Verification items for the finished model (mm, model axes). A direction names the side the tool comes from. Give positions to 0.01 mm unless a question says otherwise; leave off trailing zeros. Write each loop counter-clockwise with the first axis right and the second up, starting at its lowest first coordinate (ties: lowest second). Pieces come first, ordered by that corner, then holes. Notation, with made-up numbers: (-20, 22.5) - (-1, 22.5) arc R18 ccw to (-1, 45.5) - close; hole circle Ø11 at (23.25, 16.25). An arc over 180 degrees is marked (long way). Put each result on its own line as item: value.
Autodesk Inventor part; units mm, degrees
ref_plane "GUS_4500_1_XY" through (7.5, 20, 0) normal (1, 0, 0) x (0, 0, -1)
ref_plane "GUS_4500_1_YZ" through (7.5, 20, 0) normal (0, 0, -1) x (0, 1, 0)
ref_plane "GUS_4500_1_ZX" through (7.5, 20, 0) normal (0, 1, 0) x (1, 0, 0)
sketch "Skizze_1" plane through (0, 0, 0) normal (0, 0, 1) x (1, 0, 0)
  line L0 (0, 0) -> (40, 0)
  line L1 (40, 0) -> (40, 5.8)
  line L2 (40, 5.8) -> (18.3181, 18.3181)
  line L3 (18.3181, 18.3181) -> (5.8, 40)
  line L4 (5.8, 40) -> (0, 40)
  line L5 (0, 40) -> (0, 0)
extrude "Extrusion1" add sketch "Skizze_1" along normal mid plane 37
sketch "Skizze_2" plane through (0, 0, 0) normal (0, 0, 1) x (1, 0, 0)
  line L0 (7.5, 7.5) -> (40, 7.5)
  line L1 (40, 7.5) -> (40, 40)
  line L2 (40, 40) -> (7.5, 40)
  line L3 (7.5, 40) -> (7.5, 7.5)
extrude "Extrusion2" cut sketch "Skizze_2" along normal mid plane 25
sketch "Skizze_3" plane through (0, 0, 0) normal (0, 1, 0) x (-1, 0, 0)
  arc A0 (-20.3, -4.5) -> (-20.3, 4.5) centre (-20.3, 0) ccw
  line L0 (-20.3, 4.5) -> (-25.3, 4.5)
  arc A1 (-25.3, 4.5) -> (-25.3, -4.5) centre (-25.3, 0) ccw
  line L1 (-25.3, -4.5) -> (-20.3, -4.5)
extrude "Extrusion3" cut sketch "Skizze_3" along normal blind 7.5
sketch "Skizze_4" plane through (0, 0, 0) normal (1, 0, 0) x (0, 1, 0)
  arc A0 (20.3, 4.5) -> (20.3, -4.5) centre (20.3, 0) ccw
  line L0 (20.3, -4.5) -> (25.3, -4.5)
  arc A1 (25.3, -4.5) -> (25.3, 4.5) centre (25.3, 0) ccw
  line L1 (25.3, 4.5) -> (20.3, 4.5)
extrude "Extrusion4" cut sketch "Skizze_4" along normal blind 7.5
sketch "Skizze_5" plane through (0, 0, 0) normal (1, 0, 0) x (0, 1, 0)
  line L0 (13, 7) -> (13, -7)
  line L1 (13, -7) -> (32, -7)
  line L2 (32, -7) -> (32, 7)
  line L3 (32, 7) -> (13, 7)
extrude "Extrusion5" cut sketch "Skizze_5" along normal blind 2
sketch "Skizze_6" plane through (0, 0, 0) normal (0, 1, 0) x (-1, 0, 0)
  line L0 (-13, 7) -> (-32, 7)
  line L1 (-32, 7) -> (-32, -7)
  line L2 (-32, -7) -> (-13, -7)
  line L3 (-13, -7) -> (-13, 7)
extrude "Extrusion6" cut sketch "Skizze_6" along normal blind 2
ref_plane "GUS_4500_1_XY" through (7.5, 20, 0) normal (1, 0, 0) x (0, 0, -1)
ref_plane "GUS_4500_1_YZ" through (7.5, 20, 0) normal (0, 0, -1) x (0, 1, 0)
ref_plane "GUS_4500_1_ZX" through (7.5, 20, 0) normal (0, 1, 0) x (1, 0, 0)
ref_plane "GUS_4500_12_XY" through (7.5, 25, 0) normal (1, 0, 0) x (0, 0, -1)
ref_plane "GUS_4500_12_YZ" through (7.5, 25, 0) normal (0, 0, -1) x (0, 1, 0)
ref_plane "GUS_4500_12_ZX" through (7.5, 25, 0) normal (0, 1, 0) x (1, 0, 0)
ref_plane "GUS_4500_2_XY" through (25, 7.5, 0) normal (0, 1, 0) x (1, 0, 0)
ref_plane "GUS_4500_2_YZ" through (25, 7.5, 0) normal (1, 0, 0) x (0, 0, -1)
ref_plane "GUS_4500_2_ZX" through (25, 7.5, 0) normal (0, 0, -1) x (0, 1, 0)
ref_plane "GUS_4500_23_XY" through (20, 7.5, 0) normal (0, 1, 0) x (1, 0, 0)
ref_plane "GUS_4500_23_YZ" through (20, 7.5, 0) normal (1, 0, 0) x (0, 0, -1)
ref_plane "GUS_4500_23_ZX" through (20, 7.5, 0) normal (0, 0, -1) x (0, 1, 0)
ref_plane "p1_XY" through (0, 20, -18.5) normal (0, 0, -1) x (0, 1, 0)
ref_plane "p1_YZ" through (0, 20, -18.5) normal (0, 1, 0) x (1, 0, 0)
ref_plane "p1_ZX" through (0, 20, -18.5) normal (1, 0, 0) x (0, 0, -1)
properties part number "GUS_4501_1"
Q1. Section check A-A, the plane y = 3.5. Record the cut outline in (x, z), plus the area to 3 significant figures.
Answers follow:
outline: (0, -18.5) - (40, -18.5) - (40, 18.5) - (0, 18.5) - close; hole (20.3, -4.5) - (25.3, -4.5) arc R4.5 ccw to (25.3, 4.5) - (20.3, 4.5) arc R4.5 ccw to start
area: 1,370 mm2
Q2. Release check for a two-part mould opening along Y. For faces 1 (the face through (20, 0, -8)), 2 (the face through (3, 40, 0)), 3 (the face through (15, 16, -18.5)), 4 (the face through (4.7, 29.8, 0.1)) record: released by +Y, released by -Y, zero draft, split by the parting line, or undercut.
Answers follow:
face 1: released by -Y
face 2: released by +Y
face 3: zero draft
face 4: undercut
Q3. Section check C-C, the plane x = 19. Record the cut outline in (y, z), plus the area to 3 significant figures.
Answers follow:
outline: (0, -18.5) - (17.92, -18.5) - (17.92, -12.5) - (7.5, -12.5) - (7.5, -4.31) - (2, -4.31) - (2, -7) - (0, -7) - close; (0, 7) - (2, 7) - (2, 4.31) - (7.5, 4.31) - (7.5, 12.5) - (17.92, 12.5) - (17.92, 18.5) - (0, 18.5) - close
area: 327 mm2
Q4. Section check B-B, the plane z = 0. Record the cut outline in (x, y), plus the area to 3 significant figures.
Answers follow:
outline: (0, 0) - (13, 0) - (13, 2) - (15.8, 2) - (15.8, 7.5) - (7.5, 7.5) - (7.5, 15.8) - (2, 15.8) - (2, 13) - (0, 13) - close; (0, 32) - (2, 32) - (2, 29.8) - (7.5, 29.8) - (7.5, 37.06) - (5.8, 40) - (0, 40) - close; (29.8, 2) - (32, 2) - (32, 0) - (40, 0) - (40, 5.8) - (37.06, 7.5) - (29.8, 7.5) - close
area: 309 mm2
Q5. Scan lines: line 1 along X through (y, z) = (18.5, 4.5); line 2 along Y through (x, z) = (13, 11.5); line 3 along Z through (x, y) = (11, 10.5). Record each from-to range of solid material in increasing order.
Answers follow:
line 1: x = 2 to 7.5
line 2: y = 0 to 7.5
line 3: z = -18.5 to -12.5, 12.5 to 18.5
Q6. Go/stop test with flat-tipped pins: pin 1 Ø8 at (x, z) = (21, -1) entering from +Y; pin 2 Ø2 at (x, z) = (27.5, -13.5) entering from +Y; pin 3 Ø15 at (x, y) = (25.5, 28) entering from +Z; pin 4 Ø7.5 at (y, z) = (25.5, 5) entering from +X. Record where each tip stops, or that it passes through.
Answers follow:
pin 1: stops at y = 7.5
pin 2: stops at y = 13.59
pin 3: passes through
pin 4: stops at x = 7.5
Q7. Section check D-D, the plane z = 9.5. Record the cut outline in (x, y).
Answers follow:
outline: (0, 0) - (40, 0) - (40, 5.8) - (37.06, 7.5) - (7.5, 7.5) - (7.5, 37.06) - (5.8, 40) - (0, 40) - close
Q8. Set-up check for faces 5 (the face through (5, 23, 4.5)), 6 (the face through (16, 16, 12.5)), 7 (the face through (1, 22, -7)), 8 (the face through (13, 1, 0)): record each of +Z, -Z, +X, -X, +Y, -Y from which the full face is reachable in a straight line by a thin tool's end or side.
Answers follow:
face 5: +X, -X
face 6: +X, +Y
face 7: -X
face 8: -Y
